Could you check a few things on this model? Use its own coordinates, in mm. Face numbers are marked on the shaded views. A direction names the side the tool comes from. Give positions to 0.01 mm unless a question says otherwise; leave off trailing zeros. Write each loop counter-clockwise with the first axis right and the second up, starting at its lowest first coordinate (ties: lowest second). Pieces come first, ordered by that corner, then holes. Notation, with made-up numbers: M -37.75,-30 L 12.25,-30 A30 cw 12.25,2 Z; hole C 43,82 d6. An arc over 180 degrees is marked long. One line per item, written item: value.
```python
from build123d import *

# Parameters (mm, degrees)
F0_W      = 55
F0_H      = 55
F1_DEPTH  = 3
F2_R      = 3.5
F3_DEPTH  = 3
F4_R      = 2.9
F5_DEPTH  = 3
F6_R      = 4.5
F7_DEPTH  = 5
F8_R      = 3.25
F9_DEPTH  = 25
F10_R     = 4
F12_DEPTH = 25
F13_R     = 3
F15_DEPTH = 3
F17_DEPTH = 20


with BuildPart() as f1:
    # F0 (on Top) → F1 (new body)
    with BuildSketch(Plane.XY):
        Rectangle(F0_W, F0_H)
    extrude(amount=F1_DEPTH)

    # F2 (on face) → F3 (join)
    with BuildSketch(Plane.XY.offset(3)):
        with Locations((-15.9099025767, 15.9099025767)):
            Circle(F2_R)
        with Locations((15.9099025767, 15.9099025767)):
            Circle(F2_R)
        with Locations((-15.9099025767, -15.9099025767)):
            Circle(F2_R)
        with Locations((15.9099025767, -15.9099025767)):
            Circle(F2_R)
    extrude(amount=F3_DEPTH)

    # F4 (on face) → F5 (join)
    with BuildSketch(Plane.XY.offset(6)):
        with Locations((-15.9099025767, 15.9099025767)):
            Circle(F4_R)
        with Locations((15.9099025767, 15.9099025767)):
            Circle(F4_R)
        with Locations((-15.9099025767, -15.9099025767)):
            Circle(F4_R)
        with Locations((15.9099025767, -15.9099025767)):
            Circle(F4_R)
    extrude(amount=F5_DEPTH)

    # F6 (on face) → F7 (join, symmetric)
    with BuildSketch(Plane.XY.offset(3)):
        with Locations((-22.627416998, 22.627416998)):
            Circle(F6_R)
        with Locations((22.627416998, 22.627416998)):
            Circle(F6_R)
        with Locations((22.627416998, -22.627416998)):
            Circle(F6_R)
        with Locations((-22.627416998, -22.627416998)):
            Circle(F6_R)
    extrude(amount=F7_DEPTH, both=True)

    # F8 (on face) → F9 (cut, symmetric)
    with BuildSketch(Plane(origin=(0, 0, -2), x_dir=(1, 0, 0), z_dir=(0, 0, -1))):
        with Locations((-22.627416998, 22.627416998)):
            Circle(F8_R)
        with Locations((22.627416998, 22.627416998)):
            Circle(F8_R)
        with Locations((-22.627416998, -22.627416998)):
            Circle(F8_R)
        with Locations((22.627416998, -22.627416998)):
            Circle(F8_R)
    extrude(amount=F9_DEPTH, both=True, mode=Mode.SUBTRACT)

    # F10
    f10_edges = [f1.edges().sort_by_distance(p)[0] for p in [
        (27.5, -27.5, 1.5),
        (-27.5, -27.5, 1.5),
        (-27.5, 27.5, 1.5),
        (27.5, 27.5, 1.5),
    ]]
    fillet(f10_edges, radius=F10_R)

    # F11 (on face) → F12 (cut, symmetric)
    with BuildSketch(Plane.XY.offset(3)):
        Polygon((-12.5, 2.5), (-27.5, 17.5), (-27.5, -17.5), (-12.5, -2.5), align=None)
        Polygon((-2.5, -12.5), (-17.5, -27.5), (17.5, -27.5), (2.5, -12.5), align=None)
        Polygon((12.5, -2.5), (27.5, -17.5), (27.5, 17.5), (12.5, 2.5), align=None)
        Polygon((2.5, 12.5), (17.5, 27.5), (-17.5, 27.5), (-2.5, 12.5), align=None)
    extrude(amount=F12_DEPTH, both=True, mode=Mode.SUBTRACT)

    # F13
    f13_edges = [f1.edges().sort_by_distance(p)[0] for p in [
        (27.5, 17.5, 1.5),
        (12.5, 2.5, 1.5),
        (27.5, -17.5, 1.5),
        (17.5, -27.5, 1.5),
        (-17.5, -27.5, 1.5),
        (-2.5, -12.5, 1.5),
        (2.5, -12.5, 1.5),
        (-27.5, -17.5, 1.5),
        (-12.5, -2.5, 1.5),
        (-12.5, 2.5, 1.5),
        (-27.5, 17.5, 1.5),
        (-17.5, 27.5, 1.5),
        (-2.5, 12.5, 1.5),
        (2.5, 12.5, 1.5),
        (17.5, 27.5, 1.5),
        (12.5, -2.5, 1.5),
    ]]
    fillet(f13_edges, radius=F13_R)

    # F14 (on face) → F15 (join)
    with BuildSketch(Plane.XY.offset(3)):
        with BuildLine():
            ThreePointArc((-26.6213203436, 16.6213203436), (-27.2716385975, 17.59459039), (-27.5, 18.7426406871))
            Line((-27.5, 18.7426406871), (-27.5, -18.7426406871))
            ThreePointArc((-27.5, -18.7426406871), (-27.2716385975, -17.59459039), (-26.6213203436, -16.6213203436))
            Line((-26.6213203436, -16.6213203436), (-23.9688763441, -13.9688763441))
            Line((-23.9688763441, -13.9688763441), (-24.0687389298, 14.0687389298))
            Line((-24.0687389298, 14.0687389298), (-26.6213203436, 16.6213203436))
        make_face()
        with BuildLine():
            Line((18.7426406871, 27.5), (-18.7426406871, 27.5))
            ThreePointArc((-18.7426406871, 27.5), (-17.59459039, 27.2716385975), (-16.6213203436, 26.6213203436))
            Line((-16.6213203436, 26.6213203436), (-13.9688763441, 23.9688763441))
            Line((-13.9688763441, 23.9688763441), (14.0687389298, 24.0687389298))
            Line((14.0687389298, 24.0687389298), (16.6213203436, 26.6213203436))
            ThreePointArc((16.6213203436, 26.6213203436), (17.59459039, 27.2716385975), (18.7426406871, 27.5))
        make_face()
        with BuildLine():
            Line((27.5, -18.7426406871), (27.5, 18.7426406871))
            ThreePointArc((27.5, 18.7426406871), (27.2716385975, 17.59459039), (26.6213203436, 16.6213203436))
            Line((26.6213203436, 16.6213203436), (23.9688763441, 13.9688763441))
            Line((23.9688763441, 13.9688763441), (24.0687389298, -14.0687389298))
            Line((24.0687389298, -14.0687389298), (26.6213203436, -16.6213203436))
            ThreePointArc((26.6213203436, -16.6213203436), (27.2716385975, -17.59459039), (27.5, -18.7426406871))
        make_face()
        with BuildLine():
            ThreePointArc((-16.6213203436, -26.6213203436), (-17.59459039, -27.2716385975), (-18.7426406871, -27.5))
            Line((-18.7426406871, -27.5), (18.7426406871, -27.5))
            ThreePointArc((18.7426406871, -27.5), (17.59459039, -27.2716385975), (16.6213203436, -26.6213203436))
            Line((16.6213203436, -26.6213203436), (13.9688763441, -23.9688763441))
            Line((13.9688763441, -23.9688763441), (-14.0687389298, -24.0687389298))
            Line((-14.0687389298, -24.0687389298), (-16.6213203436, -26.6213203436))
        make_face()
    extrude(amount=-F15_DEPTH)

    # F16 (on face) → F17 (cut, symmetric)
    with BuildSketch(Plane.XY.offset(3)):
        Polygon((-27.9307178569, 26.5165042945), (-25.1022907321, 23.6880771697), (-23.6880771697, 25.1022907321), (-26.5165042945, 27.9307178569), align=None)
        Polygon((-23.6880771697, -25.1022907321), (-25.1022907321, -23.6880771697), (-27.9307178569, -26.5165042945), (-26.5165042945, -27.9307178569), align=None)
        Polygon((25.1022907321, -23.6880771697), (23.6880771697, -25.1022907321), (26.5165042945, -27.9307178569), (27.9307178569, -26.5165042945), align=None)
        Polygon((23.6880771697, 25.1022907321), (25.1022907321, 23.6880771697), (27.9307178569, 26.5165042945), (26.5165042945, 27.9307178569), align=None)
    extrude(amount=F17_DEPTH, both=True, mode=Mode.SUBTRACT)


solid = f1.part
```
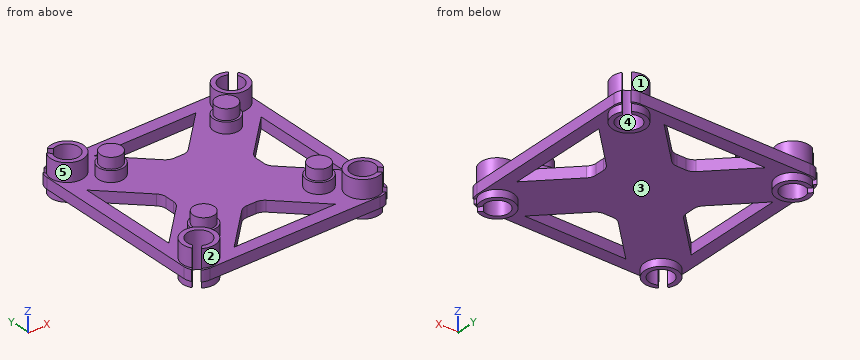
1) We'd pull the mould along X, two halves only. Please class the marked faces 1 and 2: pulls with the +X half, pulls with the -X half, needs draft (parallel to the pull), parting line crosses it, or undercut.
Outcome:
face 1: undercut
face 2: undercut
2) If we section it at B-B, the plane x = -8: Write out the boundary of the cut face in (y, z), then the cut area to 3 significant figures.
Outcome:
outline: M -27.5,0 L -24.05,0 L -24.05,3 L -27.5,3 Z; M -18,0 L 18,0 L 18,3 L -18,3 Z; M 23.99,0 L 27.5,0 L 27.5,3 L 23.99,3 Z
area: 129 mm^2
3) If we section it at A-A, the plane y = -22.5: Give the number of separate pieces and of enclosed holes in the cut face, then the cut area to 3 significant figures.
Outcome:
separate pieces: 4
enclosed holes: 0
area: 86.0 mm^2
4) On a 3-axis mill with a long thin cutter (end or side, diameter ignored), from which of +Z, -Z, +X, -X, +Y, -Y can I reach the whole of each face in a straight line? I mean the marked faces 3, 4 and 5. Say none if no direction works.
Outcome:
face 3: -Z
face 4: +Z, -Z
face 5: +Z
5) Please list where these lines run through material, in increasing order: L1, parallel to X at y = -7.5, z = 1.5; L2, parallel to X at y = -1, z = 2.75; L3, parallel to Y at x = 15, z = 0.25. Write a range as from..to.
Outcome:
L1: x = -27.5..-23.99, -17.5..17.5, 24.05..27.5
L2: x = -27.5..-24.02, -12.5..12.5, 24.02..27.5
L3: y = -27.5..-5, 5..27.5
6) If we section it at D-D, the plane y = -6.5: Write out the boundary of the cut face in (x, z).
Outcome:
outline: M -27.5,0 L -24,0 L -24,3 L -27.5,3 Z; M -16.5,0 L 16.5,0 L 16.5,3 L -16.5,3 Z; M 24.04,0 L 27.5,0 L 27.5,3 L 24.04,3 Z
7) If we section it at C-C, the plane z = 7: Write out the boundary of the cut face in (x, y), then the cut area to 3 significant figures.
Outcome:
outline: M -26.44,-25.02 L -25.52,-24.11 A3.25 cw long -24.11,-25.52 L -25.02,-26.44 A4.5 ccw long Z; M -26.44,25.02 A4.5 ccw long -25.02,26.44 L -24.11,25.52 A3.25 cw long -25.52,24.11 Z; C -15.91,-15.91 d5.8; C -15.91,15.91 d5.8; C 15.91,-15.91 d5.8; C 15.91,15.91 d5.8; M 24.11,-25.52 A3.25 cw long 25.52,-24.11 L 26.44,-25.02 A4.5 ccw long 25.02,-26.44 Z; M 24.11,25.52 L 25.02,26.44 A4.5 ccw long 26.44,25.02 L 25.52,24.11 A3.25 cw long Z
area: 217 mm^2
8) I'm going to push flat-ended pins straight in: pin 1 (2 mm diameter, centred on y = 15.5, z = 6.5, fed in from +X); pin 2 (7.5 mm diameter, centred on x = 22.63, y = 22.63, fed in from +Z); pin 3 (1 mm diameter, centred on x = 18.5, z = 4, fed in from +Y). Where does each tip first touch, or does it pass through?
Outcome:
pin 1: stops at x = 19.41
pin 2: stops at z = 8
pin 3: stops at y = 25.29
